```python
from build123d import *

# Parameters (mm, degrees)
SKETCH1_W            = 63.5
SKETCH1_H            = 33.401
SKETCH1_W_2          = 10.16
SKETCH1_H_2          = 3.175
SKETCH1_W_3          = 40.64
SKETCH1_H_3          = 20.066
MAIN_EXTRUSION_DEPTH = 3.175
SKETCH3_R            = 2.2225
MOUNTING_HOLES_DEPTH = 37.777630008
TAB_CUTOUT_DEPTH     = 37.777630008
FILLET1_R            = 5.08


with BuildPart() as part:
    # Sketch1 → Main Extrusion (new body)
    with BuildSketch(Plane(origin=(0, 0, 0), x_dir=(1, 0, 0), z_dir=(0, 1, 0))):
        with Locations((0, 1.5875)):
            Rectangle(SKETCH1_W, SKETCH1_H)
        with Locations((21.59, 14.1605)):
            Rectangle(SKETCH1_W_2, SKETCH1_H_2, mode=Mode.SUBTRACT)
        with Locations((1.27, 14.1605)):
            Rectangle(SKETCH1_W_2, SKETCH1_H_2, mode=Mode.SUBTRACT)
        with Locations((-19.05, 14.1605)):
            Rectangle(SKETCH1_W_2, SKETCH1_H_2, mode=Mode.SUBTRACT)
        Rectangle(SKETCH1_W_3, SKETCH1_H_3, mode=Mode.SUBTRACT)
    extrude(amount=MAIN_EXTRUSION_DEPTH)

    # Sketch3 → Mounting Holes (cut, through all)
    with BuildSketch(Plane(origin=(0, 3.175, 0), x_dir=(1, 0, 0), z_dir=(0, 1, 0))):
        with Locations(Location((-24.357246486, 4.9657, 0), (0, 0, 270))):
            Circle(SKETCH3_R)
        with Locations(Location((-24.357246486, -4.9657, 0), (0, 0, 270))):
            Circle(SKETCH3_R)
        with Locations(Location((24.357246486, -4.9657, 0), (0, 0, 90))):
            Circle(SKETCH3_R)
        with Locations(Location((24.357246486, 4.9657, 0), (0, 0, 90))):
            Circle(SKETCH3_R)
    extrude(amount=-MOUNTING_HOLES_DEPTH, mode=Mode.SUBTRACT)

    # Sketch5 → Tab cutout (cut, through all)
    with BuildSketch(Plane(origin=(0, 3.175, 0), x_dir=(1, 0, 0), z_dir=(0, 1, 0))):
        Polygon((-20.32, 0), (-20.32, 0.889), (-27.305, 0.889), (-27.305, -0.889), (-20.32, -0.889), align=None)
        Polygon((27.305, -0.889), (20.32, -0.889), (20.32, 0), (20.32, 0.889), (27.305, 0.889), align=None)
    extrude(amount=-TAB_CUTOUT_DEPTH, mode=Mode.SUBTRACT)

    # Fillet1
    fillet1_edges = [part.edges().sort_by_distance(p)[0] for p in [
        (31.75, 1.5875, 15.113),
        (-31.75, 1.5875, 15.113),
        (-31.75, 1.5875, -18.288),
        (31.75, 1.5875, -18.288),
    ]]
    fillet(fillet1_edges, radius=FILLET1_R)


solid = part.part
```
Could you check a few things on this model? Use its own coordinates, in mm. A direction names the side the tool comes from. Coordinates: 2 decimals unless noted, no trailing zeros. Write each loop counter-clockwise with the first axis right and the second up, starting at its lowest first coordinate (ties: lowest second). Pieces come first, ordered by that corner, then holes. Notation, with made-up numbers: (60, 72) - (80, 72) arc R11 ccw to (80, 82) - close; hole circle Ø1 at (23, 53.25). An arc over 180 degrees is marked (long way). Use a Markdown table: item, result.
Q1. Please list where these lines run through material, in increasing order: L1, parallel to Z at x = 20, y = 1.9; L2, parallel to Z at x = 24.5, y = 1.55; L3, parallel to Z at x = -11.5, y = 1.
Geometry check:
| item | result |
|---|---|
| L1 | z = -18.29 to -15.75, -12.57 to -10.03, 10.03 to 15.11 |
| L2 | z = -18.29 to -15.75, -12.57 to -7.18, -2.75 to -0.89, 0.89 to 2.75, 7.18 to 15.11 |
| L3 | z = -18.29 to -10.03, 10.03 to 15.11 |
Q2. I'm going to push a flat-ended pin straight in: pin 1 Ø1.6 at (y, z) = (1, -15) entering from +X. Where does the tip first touch, or does it pass through?
Geometry check:
| item | result |
|---|---|
| pin 1 | stops at x = 31.65 |
Q3. Imagine slicing it at A-A (x = 10.5). List the corners of the cut face in (y, z) for me (3 decimals), and give its area (3 significant figures).
Geometry check:
| item | result |
|---|---|
| outline | (0, -18.288) - (3.175, -18.288) - (3.175, -10.033) - (0, -10.033) - close; (0, 10.033) - (3.175, 10.033) - (3.175, 15.113) - (0, 15.113) - close |
| area | 42.3 mm2 |
Q4. Imagine slicing it at B-B (x = -15). List the corners of the cut face in (y, z) for me (3 decimals).
Geometry check:
| item | result |
|---|---|
| outline | (0, -18.288) - (3.175, -18.288) - (3.175, -15.748) - (0, -15.748) - close; (0, -12.573) - (3.175, -12.573) - (3.175, -10.033) - (0, -10.033) - close; (0, 10.033) - (3.175, 10.033) - (3.175, 15.113) - (0, 15.113) - close |
Q5. Imagine slicing it at D-D (x = -23.5). List the corners of the cut face in (y, z) for me (3 decimals).
Geometry check:
| item | result |
|---|---|
| outline | (0, -18.288) - (3.175, -18.288) - (3.175, -15.748) - (0, -15.748) - close; (0, -12.573) - (3.175, -12.573) - (3.175, -7.016) - (0, -7.016) - close; (0, -2.915) - (3.175, -2.915) - (3.175, -0.889) - (0, -0.889) - close; (0, 0.889) - (3.175, 0.889) - (3.175, 2.915) - (0, 2.915) - close; (0, 7.016) - (3.175, 7.016) - (3.175, 15.113) - (0, 15.113) - close |
Q6. Which directions (+Z, -Z, +X, -X, +Y, -Y) give clear straight access to the entire face, cutting with the end or side of a thin tool? Please do faces 1 (the flat face through (31.75, 2, -1)), 2 (the flat face through (27.305, 2, 0)).
Geometry check:
| item | result |
|---|---|
| face 1 | +Z, -Z, +X, +Y, -Y |
| face 2 | +Y, -Y |
Q7. Thinking about a two-plate mould opening in Z: for faces 3 (the flat face through (20.32, 2, -5)), 4 (the cylindrical face through (-30.3, 1.61, -16.76)), 5 (the flat face through (-31.75, 2, -1)), which applies, +Z half, -Z half, draft (parallel to the pull), parting line (faces both ways), or undercut?
Geometry check:
| item | result |
|---|---|
| face 3 | undercut |
| face 4 | -Z half |
| face 5 | draft |
Q8. Imagine slicing it at C-C (z = 6.5). List the corners of the cut face in (x, y) for me (3 decimals), and give its area (3 significant figures).
Geometry check:
| item | result |
|---|---|
| outline | (-31.75, 0) - (-25.965, 0) - (-25.965, 3.175) - (-31.75, 3.175) - close; (-22.749, 0) - (-20.32, 0) - (-20.32, 3.175) - (-22.749, 3.175) - close; (20.32, 0) - (22.749, 0) - (22.749, 3.175) - (20.32, 3.175) - close; (25.965, 0) - (31.75, 0) - (31.75, 3.175) - (25.965, 3.175) - close |
| area | 52.2 mm2 |
